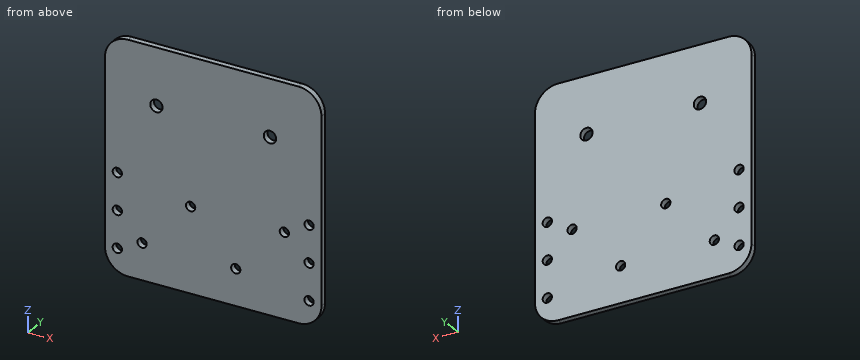
```python
from build123d import *

# Parameters (mm, degrees)
SKETCH1_W           = 70
SKETCH1_H           = 75
SKETCH1_R           = 1.5
SKETCH1_R_2         = 2
BOSS_EXTRUDE1_DEPTH = 2
FILLET2_R           = 7.5


with BuildPart() as part:
    # Sketch1 → Boss-Extrude1 (new body)
    with BuildSketch(Plane(origin=(0, 0, 0), x_dir=(1, 0, 0), z_dir=(0, 1, 0))):
        with Locations((0, -1)):
            Rectangle(SKETCH1_W, SKETCH1_H)
        with Locations(Location((7.3, 24.7, 0), (0, 0, 270))):
            Circle(SKETCH1_R, mode=Mode.SUBTRACT)
        with Locations(Location((23, 8.9, 0), (0, 0, 270))):
            Circle(SKETCH1_R, mode=Mode.SUBTRACT)
        with Locations(Location((-23, 24.7, 0), (0, 0, 270))):
            Circle(SKETCH1_R, mode=Mode.SUBTRACT)
        with Locations(Location((-7.3, 8.9, 0), (0, 0, 270))):
            Circle(SKETCH1_R, mode=Mode.SUBTRACT)
        with Locations(Location((31, 16.5, 0), (0, 0, 270))):
            Circle(SKETCH1_R, mode=Mode.SUBTRACT)
        with Locations(Location((31, 28.5, 0), (0, 0, 270))):
            Circle(SKETCH1_R, mode=Mode.SUBTRACT)
        with Locations(Location((31, 4.5, 0), (0, 0, 270))):
            Circle(SKETCH1_R, mode=Mode.SUBTRACT)
        with Locations(Location((-31, 28.5, 0), (0, 0, 90))):
            Circle(SKETCH1_R, mode=Mode.SUBTRACT)
        with Locations(Location((-31, 16.5, 0), (0, 0, 90))):
            Circle(SKETCH1_R, mode=Mode.SUBTRACT)
        with Locations(Location((-31, 4.5, 0), (0, 0, 90))):
            Circle(SKETCH1_R, mode=Mode.SUBTRACT)
        with Locations(Location((18.35, -20, 0), (0, 0, 270))):
            Circle(SKETCH1_R_2, mode=Mode.SUBTRACT)
        with Locations(Location((-18.35, -20, 0), (0, 0, 90))):
            Circle(SKETCH1_R_2, mode=Mode.SUBTRACT)
    extrude(amount=BOSS_EXTRUDE1_DEPTH)

    # Fillet2
    fillet2_edges = [part.edges().sort_by_distance(p)[0] for p in [
        (-35, 1, -36.5),
        (35, 1, -36.5),
        (35, 1, 38.5),
        (-35, 1, 38.5),
    ]]
    fillet(fillet2_edges, radius=FILLET2_R)


solid = part.part
```
The listing builds one solid part. Answer for the finished solid, in the listing's coordinates (mm). Coordinates: 2 decimals unless noted, no trailing zeros. Write each loop counter-clockwise with the first axis right and the second up, starting at its lowest first coordinate (ties: lowest second). Pieces come first, ordered by that corner, then holes.
Q1. Section C-C, the plane y = 1 is taken. Give the number of separate pieces and of enclosed holes in the cut face, then the cut area to 3 significant figures.
Returned:
separate pieces: 1
enclosed holes: 12
area: 5,110 mm2
Q2. Find the intervals of material crossed by line 1 along X through (y, z) = (0.4, -16.5); line 2 along X through (y, z) = (0.5, -24.7); line 3 along Z through (x, y) = (-18.35, 1.2), in increasing order.
Returned:
line 1: x = -35 to -32.5, -29.5 to 29.5, 32.5 to 35
line 2: x = -35 to -24.5, -21.5 to 5.8, 8.8 to 35
line 3: z = -36.5 to 18, 22 to 38.5
Q3. Section D-D, the plane x = 31 is taken. Write down the section's boundary in (y, z).
Returned:
outline: (0, -35.63) - (2, -35.63) - (2, -30) - (0, -30) - close; (0, -27) - (2, -27) - (2, -18) - (0, -18) - close; (0, -15) - (2, -15) - (2, -6) - (0, -6) - close; (0, -3) - (2, -3) - (2, 37.63) - (0, 37.63) - close
Q4. Section B-B, the plane z = -8.9 is taken. Write down the section's boundary in (x, y).
Returned:
outline: (-35, 0) - (-8.8, 0) - (-8.8, 2) - (-35, 2) - close; (-5.8, 0) - (21.5, 0) - (21.5, 2) - (-5.8, 2) - close; (24.5, 0) - (35, 0) - (35, 2) - (24.5, 2) - close
Q5. Section A-A, the plane x = 18.35 is taken. Write down the section's boundary in (y, z).
Returned:
outline: (0, -36.5) - (2, -36.5) - (2, 18) - (0, 18) - close; (0, 22) - (2, 22) - (2, 38.5) - (0, 38.5) - close
